Could you check a few things on this drawing? It's one solid part, dimensions in mm from its lowest x, y, z. A direction names the side the tool comes from. Coordinates: 2 decimals unless noted, no trailing zeros. Order: outer loops, then holes, each group sorted by start corner. A loop starts at its lowest first (then second) coordinate and runs counter-clockwise, first axis right, second up. Notation, with made-up numbers: (-17, -18.75) - (-11, -18.75) arc R15 cw to (-11, 3.25) - close; hole circle Ø11 at (62.25, 72). An arc over 180 degrees is marked (long way). Return JSON: item names as keys, results as strings. Group by question number.
1) For pin 1 Ø1 at (x, z) = (82.41, 13.68) entering from -Y; pin 2 Ø6 at (x, z) = (76.5, 17.5) entering from +Y, each with a flat end and sliding along its axis, tell me the tip position at first contact or that it passes through.
2) Imagine slicing it at A-A (y = 13). Write out the boundary of the cut face in (x, z), and give its area (3 significant figures).
3) If we mould it in two halves opening along Z, with no side actions, what happens to the marked faces 1, 2 and 3? For each: pulls with the +Z half, pulls with the -Z half, needs draft (parallel to the pull), parting line crosses it, or undercut.
4) Which directions (+Z, -Z, +X, -X, +Y, -Y) give clear straight access to the entire face, cutting with the end or side of a thin tool? Please do the marked faces 4 and 5.
5) If I drill on line 1 along X through (y, z) = (1.5, 11.5) (1 decimal); line 2 along X through (y, z) = (5.5, 15); line 3 along Z through (x, y) = (18, 3.25), over which ranges is the centre line in solid material (lowest first)?
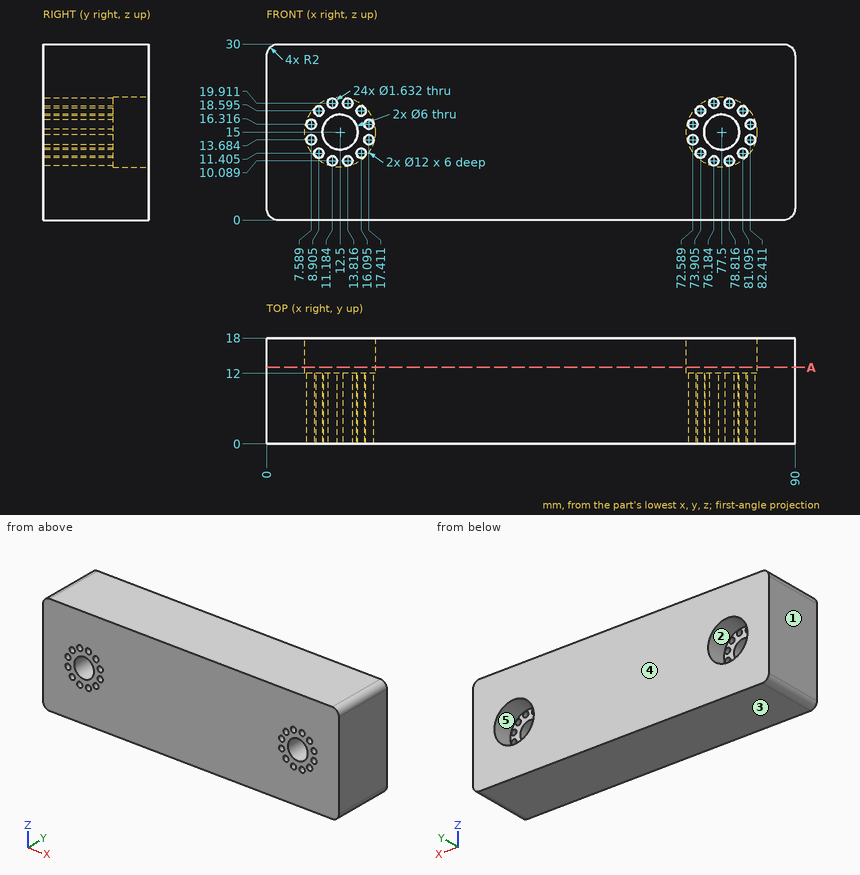
Calculated:
{
 "1": {"pin 1": "through", "pin 2": "y = 12"},
 "2": {"outline": "(0, 2) arc R2 ccw to (2, 0) - (88, 0) arc R2 ccw to (90, 2) - (90, 28) arc R2 ccw to (88, 30) - (2, 30) arc R2 ccw to (0, 28) - close; hole circle Ø12 at (12.5, 15); hole circle Ø12 at (77.5, 15)", "area": "2,470 mm2"},
 "3": {"face 1": "needs draft", "face 2": "undercut", "face 3": "pulls with the -Z half"},
 "4": {"face 4": "+Z, -Z, +X, -X, +Y", "face 5": "+Y"},
 "5": {"line 1": "0 to 8.1, 9.7 to 15.3, 16.9 to 73.1, 74.7 to 80.3, 81.9 to 90", "line 2": "0 to 9.5, 15.5 to 74.5, 80.5 to 90", "line 3": "0 to 13.12, 14.25 to 15.75, 16.88 to 30"}
}
